For this review, take the finished solid that the model builds, in its own axes (mm). A direction names the side the tool comes from. Round coordinates to 2 decimals unless told otherwise and drop trailing zeros. Loops run counter-clockwise (first coordinate to the right, second up) from the corner with the lowest first, then second, coordinate; pieces in that order, holes last.
1. To check wall thickness, follow line 1 along X through (y, z) = (-16, 18.5); line 2 along X through (y, z) = (-9.5, -13) (3 decimals); line 3 along X through (y, z) = (-8, -2) (3 decimals). State the ranges of each line that lie inside material, in increasing order.
2. Consider section C-C on x = 299. State the section outline as (y, z) points, then the cut area to 3 significant figures.
3. Draft analysis for pull direction X (two halves, no side actions). For faces 6 (the flat face through (23.339, 0.146, 21.293)), 7 (the cylindrical face through (340.942, 11.398, -14.865)), 8 (the flat face through (371, -10.16, 0)), state which applies: released by +X, released by -X, zero draft, split by the parting line, or undercut.
4. Consider section B-B on x = 20.32. State the section outline as (y, z) points, then the cut area to 3 significant figures.
5. Consider section D-D on z = 4. State how many separate pieces and enclosed holes the cut face has, then the cut area to 3 significant figures.
6. Tool access review of faces 1 (the flat face through (23.148, 0.146, -21.256)), 2 (the flat face through (35.56, -16, 0)), 3 (the flat face through (337.185, 8, 4)), 4 (the flat face through (13.6, 10.414, 4.9)), 5 (the cylindrical face through (12.749, 0.146, 2.384)): name each direction out of +Z, -Z, +X, -X, +Y, -Y from which nothing blocks a thin tool from reaching the whole face with its end or side.
7. Consider section A-A on y = 0. State the section outline as (x, z) points (1 decimal).
8. Clearance check with flat-ended pins moving along their axes: pin 1 Ø20.5 at (x, z) = (20.32, 0) entering from +Y; pin 2 Ø8 at (x, y) = (79.5, 16) entering from +Z; pin 3 Ø1 at (x, z) = (159, 18.5) entering from -Y. State where each tip first meets the part, or that it passes through.
from build123d import *

# Parameters (mm, degrees)
F2_W      = 38.1
F2_H      = 63.5
F3_DEPTH  = 35.56
F4_R      = 7.9375
F5_DEPTH  = 20.828
F6_W      = 25.4
F6_H      = 25.4
F7_DEPTH  = 44.704
F8_R      = 18.542
F9_DEPTH  = 20.32
F11_DEPTH = 12.7
F13_DEPTH = 25.4
F15_DEPTH = 25.4
F16_R     = 7.9375
F17_DEPTH = 35.942


with BuildPart() as f1:
    # F0 (on Front) → F1 (revolve)
    with BuildSketch(Plane.XZ):
        Polygon((232.41, 25.781), (0, 25.781), (0, 0), (409.829, 0), (409.829, 14.605), (347.599, 14.605), (344.805, 18.7325), (337.185, 18.7325), (337.185, 8.001), (232.41, 8.001), align=None)
    revolve(axis=Axis((144.6166912608, 0, 0), (1, 0, 0)))

    # F2 (on face) → F3 (cut)
    with BuildSketch(Plane(origin=(0, 0, 0), x_dir=(0, -1, 0), z_dir=(-1, 0, 0))):
        with Locations((29.464, 0)):
            Rectangle(F2_W, F2_H)
        with Locations((-29.464, 0)):
            Rectangle(F2_W, F2_H)
    extrude(amount=-F3_DEPTH, mode=Mode.SUBTRACT)

    # F4 (on face) → F5 (cut, through all)
    with BuildSketch(Plane(origin=(0, 10.414, 0), x_dir=(-1, 0, 0), z_dir=(0, 1, 0))):
        with BuildLine():
            Line((10.16, 25.781), (-35.56, 25.781))
            Line((-35.56, 25.781), (-30.060738686, 22.606))
            Line((-30.060738686, 22.606), (-16.4254601504, 19.9432935936))
            ThreePointArc((-16.4254601504, 19.9432935936), (0, 0), (-16.4254601504, -19.9432935936))
            Line((-16.4254601504, -19.9432935936), (-30.060738686, -22.606))
            Line((-30.060738686, -22.606), (-35.56, -25.781))
            Line((-35.56, -25.781), (10.16, -25.781))
            Line((10.16, -25.781), (10.16, 25.781))
        make_face()
        with Locations((-20.32, 0)):
            Circle(F4_R)
    extrude(amount=-F5_DEPTH, mode=Mode.SUBTRACT)

    # F6 (on face) → F7 (cut)
    with BuildSketch(Plane.YZ.offset(409.829)):
        with Locations((22.86, 0)):
            Rectangle(F6_W, F6_H)
        with Locations((-22.86, 0)):
            Rectangle(F6_W, F6_H)
    extrude(amount=-F7_DEPTH, mode=Mode.SUBTRACT)

    # F8 (on face) → F9 (join, through all)
    with BuildSketch(Plane(origin=(0, 10.16, 0), x_dir=(-1, 0, 0), z_dir=(0, 1, 0))):
        with Locations((-379.095, 0)):
            Circle(F8_R)
    extrude(amount=-F9_DEPTH)

    # F10 (on Front) → F11 (cut, symmetric)
    with BuildSketch(Plane.XZ):
        with BuildLine():
            Line((409.829, 14.605), (390.5186482351, 14.605))
            ThreePointArc((390.5186482351, 14.605), (397.637, 0), (390.5186482351, -14.605))
            Line((390.5186482351, -14.605), (409.829, -14.605))
            Line((409.829, -14.605), (409.829, 14.605))
        make_face()
    extrude(amount=F11_DEPTH, both=True, mode=Mode.SUBTRACT)

    # F12 (on face) → F13 (cut)
    with BuildSketch(Plane(origin=(0, 10.16, 0), x_dir=(-1, 0, 0), z_dir=(0, 1, 0))):
        with BuildLine():
            ThreePointArc((-365.5518286226, -12.6644491804), (-360.553, 0), (-365.5518286226, 12.6644491804))
            Line((-365.5518286226, 12.6644491804), (-365.5518286226, -12.6644491804))
        make_face()
    extrude(amount=F13_DEPTH, mode=Mode.SUBTRACT)

    # F14 (on face) → F15 (cut)
    with BuildSketch(Plane.XZ.offset(10.16)):
        with BuildLine():
            Line((365.125, -12.192), (365.125, 12.192))
            ThreePointArc((365.125, 12.192), (360.553, 0), (365.125, -12.192))
        make_face()
    extrude(amount=F15_DEPTH, mode=Mode.SUBTRACT)

    # F16 (on face) → F17 (cut, through all)
    with BuildSketch(Plane.XZ.offset(10.16)):
        with Locations((379.095, 0)):
            Circle(F16_R)
    extrude(amount=-F17_DEPTH, mode=Mode.SUBTRACT)


solid = f1.part
Resolved:
1. line 1: x = 35.56 to 232.41
1. line 2: x = 4.703 to 232.41, 337.185 to 346.586, 365.874 to 392.316
1. line 3: x = 0.099 to 12.639, 28.001 to 232.41, 337.185 to 371.414, 386.776 to 397.529
2. outline: circle Ø16 at (0, 0)
2. area: 201 mm2
3. face 6: released by -X
3. face 7: undercut
3. face 8: zero draft
4. outline: (-10.41, -20.7) - (10.41, -20.7) - (10.41, -7.94) - (-10.41, -7.94) - close; (-10.41, 7.94) - (10.41, 7.94) - (10.41, 20.7) - (-10.41, 20.7) - close
4. area: 532 mm2
5. separate pieces: 3
5. enclosed holes: 0
5. area: 13,100 mm2
6. face 1: -Z, -X, +Y, -Y
6. face 2: +Z, -Z, -X, -Y
6. face 3: none
6. face 4: +Z, -Z, -X, +Y
6. face 5: +Y, -Y
7. outline: (16.4, -19.9) - (30.1, -22.6) - (35.6, -25.8) - (232.4, -25.8) - (232.4, -8) - (337.2, -8) - (337.2, -18.7) - (344.8, -18.7) - (347.6, -14.6) - (367.7, -14.6) arc R18.5 ccw (long way) to (367.7, 14.6) - (347.6, 14.6) - (344.8, 18.7) - (337.2, 18.7) - (337.2, 8) - (232.4, 8) - (232.4, 25.8) - (35.6, 25.8) - (30.1, 22.6) - (16.4, 19.9) arc R20.3 ccw to start; hole circle Ø15.9 at (20.3, 0); hole circle Ø15.9 at (379.1, 0)
8. pin 1: stops at y = 10.41
8. pin 2: stops at z = 22.82
8. pin 3: stops at y = -18.46
